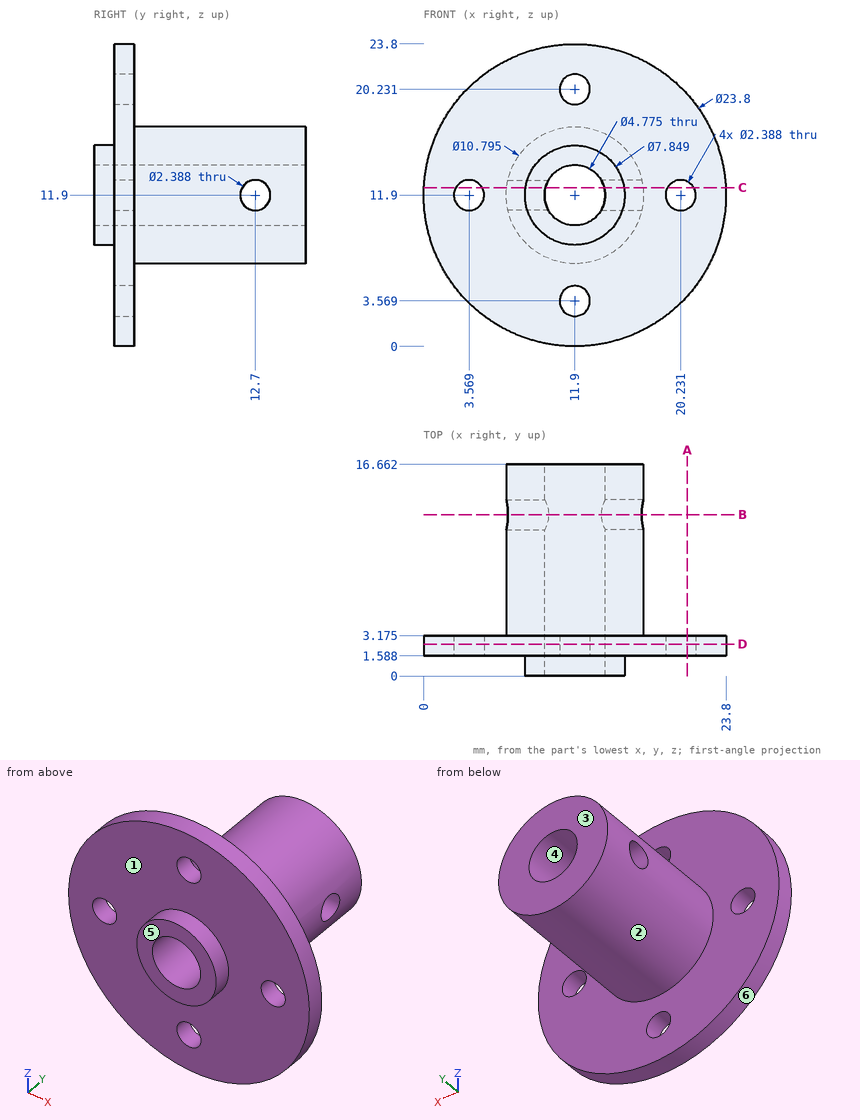
Check sheet for the drawn part. Datum: minimum x, y, z corner. Units: mm. A direction names the side the tool comes from. Coordinates: 2 decimals unless noted, no trailing zeros. Order: outer loops, then holes, each group sorted by start corner. A loop starts at its lowest first (then second) coordinate and runs counter-clockwise, first axis right, second up. Notation, with made-up numbers: M 44.5,70 L 54.5,70 A33 cw 54.5,104 Z; hole C 5,38.25 d8. An arc over 180 degrees is marked long. One line per question, with ' | ' between items. Start each with the question number.
Item 1: Sectioned sample at C-C on z = 12.5. Count the separate pieces of the cut face and the enclosed holes in it.
Item 2: Sectioned sample at A-A on x = 20.75. Record the cut outline in (y, z) (1 decimal).
Item 3: Mould release check, pull along Z, two halves, no side actions. Record for the marked faces 4, 5 and 6: pulls with the +Z half, pulls with the -Z half, needs draft (parallel to the pull), parting line crosses it, or undercut.
Item 4: Access from +Z, -Z, +X, -X, +Y, -Y to the whole of each face (thin tool, end or side, straight path). Record for the marked faces 1, 2 and 3.
Item 5: Sectioned sample at D-D on y = 2.5. Record the cut outline in (x, z) (1 decimal).
Item 6: Sectioned sample at B-B on y = 12.7. Record the cut outline in (x, z) (1 decimal).
Item 7: Gauge pin test, flat ends, axial feed: P1, Ø2.5, axis at x = 20.23, z = 11.9, coming from the -Y side; P2, Ø5, axis at x = 18.5, y = 4.5, coming from the -Z side (1 decimal); P3, Ø2, axis at x = 13, z = 3.5, coming from the +Y side (1 decimal). Record the tip position at first contact, or that the pin passes through.
Item 8: Material ranges on line 1 (X direction, y = 6.25, z = 12) (1 decimal); line 2 (Y direction, x = 15.75, z = 9.5); line 3 (Y direction, x = 22.5, z = 9) (1 decimal), recorded low to high.
Answer below:
1) separate pieces: 6 | enclosed holes: 0
2) outline: M 1.6,3.9 L 3.2,3.9 L 3.2,10.8 L 1.6,10.8 Z; M 1.6,13 L 3.2,13 L 3.2,19.9 L 1.6,19.9 Z
3) face 4: undercut | face 5: needs draft | face 6: parting line crosses it
4) face 1: -Y | face 2: +Y | face 3: +Z, -Z, +X, -X, +Y
5) outline: C 11.9,11.9 d23.8; hole C 3.6,11.9 d2.4; hole C 11.9,11.9 d4.8; hole C 11.9,3.6 d2.4; hole C 11.9,20.2 d2.4; hole C 20.2,11.9 d2.4
6) outline: M 6.6,10.7 A5.4 ccw 17.2,10.7 L 14,10.7 A2.4 cw 9.8,10.7 Z; M 6.6,13.1 L 9.8,13.1 A2.4 cw 14,13.1 L 17.2,13.1 A5.4 ccw Z
7) P1: stops at y = 1.59 | P2: stops at z = 0.9 | P3: stops at y = 3.2
8) line 1: x = 6.5 to 9.5, 14.3 to 17.3 | line 2: y = 1.59 to 16.66 | line 3: y = 1.6 to 3.2
